For this review, take the finished solid that the model builds, in its own axes (mm). A direction names the side the tool comes from. Coordinates: 2 decimals unless noted, no trailing zeros. Write each loop counter-clockwise with the first axis right and the second up, starting at its lowest first coordinate (ties: lowest second). Pieces come first, ordered by that corner, then holes.
1) We need section C-C on y = -13.5. Write out the cut boundary in (x, z), then the cut area to 3 significant figures.
2) For faces 1 (the face through (-26, -7, -5)), 2 (the face through (-26, -4, -2.5)), 3 (the face through (39.5, -9, 0)), list the 3-axis set-ups (+Z, -Z, +X, -X, +Y, -Y) from which the entire face can be reached by the end or side of a thin tool; tool diameter is ignored.
3) Mouldability with a two-part tool opening along X and no side actions: class faces 4 (the face through (-24.905, -5.456, 4.648)), 5 (the face through (-24.905, -5.456, -4.73)), 6 (the face through (41, -18, -7.52)), 7 (the face through (-42.5, -1, 0)) as pulls with the +X half, pulls with the -X half, needs draft (parallel to the pull), parting line crosses it, or undercut.
4) To check wall thickness, follow line 1 along Y through (x, z) = (-25.5, -3.8); line 2 along Y through (x, z) = (13, -15.5); line 3 along X through (y, z) = (-9.5, 6.5). State the ranges of each line that lie inside material, in increasing order.
5) We need section A-A on y = -19.1. Write out the cut boundary in (x, z).
6) Insertion check: P1, Ø8.5, axis at y = -12.5, z = -5.5, coming from the -X side; P2, Ø2, axis at x = -25.5, y = -5, coming from the +Z side; P3, Ø3, axis at x = -25.5, y = -6, coming from the -Z side. Each pin has a flat end and moves straight along its axis. Give the tip position at first contact, or say it passes through.
from build123d import *

# Parameters (mm, degrees)
SKETCH1_W                  = 85
SKETCH1_H                  = 48
BOSS_EXTRUDE1_DEPTH        = 3
SKETCH2_W                  = 3
SKETCH2_H                  = 48
BOSS_EXTRUDE2_DEPTH        = 18
M1_6_CLEARANCE_HOLE2_D     = 1.8
SKETCH11_W                 = 15.04
SKETCH11_H                 = 5
CUT_EXTRUDE5_DEPTH         = 91.785461391
SKETCH14_W                 = 10.48
SKETCH14_H                 = 18
CUT_EXTRUDE6_DEPTH         = 88.982952894
FILLET1_R                  = 1
FILLET2_R                  = 1
FILLET3_R                  = 1
FILLET4_R                  = 1
FILLET5_R                  = 1
FILLET6_R                  = 1
SKETCH17_R                 = 23
CUT_EXTRUDE11_DEPTH        = 1
FILLET9_R                  = 1
FILLET10_R                 = 10
FILLET11_R                 = 10
SKETCH18_W                 = 6
SKETCH18_H                 = 4.397787755
SKETCH18_H_2               = 4.357175314
BOSS_EXTRUDE3_DEPTH        = 4
F_1_5_1_5_DIAMETER_HOLE1_D = 1.5


with BuildPart() as part:
    # Sketch1 → Boss-Extrude1 (new body)
    with BuildSketch(Plane(origin=(0, 0, 0), x_dir=(1, 0, 0), z_dir=(0, 1, 0))):
        Rectangle(SKETCH1_W, SKETCH1_H)
    extrude(amount=-BOSS_EXTRUDE1_DEPTH)

    # Sketch2 → Boss-Extrude2 (add)
    with BuildSketch(Plane.XZ.offset(3)):
        with Locations((41, 0)):
            Rectangle(SKETCH2_W, SKETCH2_H)
    extrude(amount=BOSS_EXTRUDE2_DEPTH)

    # M1.6 Clearance Hole2 (through all)
    with Locations(Plane(origin=(0, 0, -24), x_dir=(-1, 0, 0), z_dir=(0, 0, -1))):
        with Locations((-41, -19.1)):
            Hole(M1_6_CLEARANCE_HOLE2_D / 2)

    # Sketch11 → Cut-Extrude5 (cut, through all)
    with BuildSketch(Plane(origin=(42.5, 0, 0), x_dir=(0, 0, -1), z_dir=(1, 0, 0))):
        with Locations((0, -18.5)):
            Rectangle(SKETCH11_W, SKETCH11_H)
    extrude(amount=-CUT_EXTRUDE5_DEPTH, mode=Mode.SUBTRACT)

    # Sketch14 → Cut-Extrude6 (cut, through all)
    with BuildSketch(Plane.ZY.offset(-39.5)):
        with Locations((-18.76, -12)):
            Rectangle(SKETCH14_W, SKETCH14_H)
        with Locations((18.76, -12)):
            Rectangle(SKETCH14_W, SKETCH14_H)
    extrude(amount=-CUT_EXTRUDE6_DEPTH, mode=Mode.SUBTRACT)

    # Fillet1
    fillet1_edges = [part.edges().sort_by_distance(p)[0] for p in [
        (42.5, -21, -10.52),
    ]]
    fillet(fillet1_edges, radius=FILLET1_R)

    # Fillet2
    fillet2_edges = [part.edges().sort_by_distance(p)[0] for p in [
        (42.5, -21, 10.52),
    ]]
    fillet(fillet2_edges, radius=FILLET2_R)

    # Fillet3
    fillet3_edges = [part.edges().sort_by_distance(p)[0] for p in [
        (39.5, -21, -10.52),
    ]]
    fillet(fillet3_edges, radius=FILLET3_R)

    # Fillet4
    fillet4_edges = [part.edges().sort_by_distance(p)[0] for p in [
        (39.5, -21, 10.52),
    ]]
    fillet(fillet4_edges, radius=FILLET4_R)

    # Fillet5
    fillet5_edges = [part.edges().sort_by_distance(p)[0] for p in [
        (42.5, -16, 0),
    ]]
    fillet(fillet5_edges, radius=FILLET5_R)

    # Fillet6
    fillet6_edges = [part.edges().sort_by_distance(p)[0] for p in [
        (39.5, -16, 0),
    ]]
    fillet(fillet6_edges, radius=FILLET6_R)

    # Sketch17 → Cut-Extrude11 (cut)
    with BuildSketch(Plane.XZ.offset(3)):
        with Locations(Location((2.21, 0, 0), (0, 0, 270))):
            Circle(SKETCH17_R)
    extrude(amount=-CUT_EXTRUDE11_DEPTH, mode=Mode.SUBTRACT)

    # Fillet9
    fillet9_edges = [part.edges().sort_by_distance(p)[0] for p in [
        (2.21, -3, 23),
    ]]
    fillet(fillet9_edges, radius=FILLET9_R - 0.0001)  # a hair under: the kernel refuses the full size

    # Fillet10
    fillet10_edges = [part.edges().sort_by_distance(p)[0] for p in [
        (-42.5, -1.5, -24),
    ]]
    fillet(fillet10_edges, radius=FILLET10_R)

    # Fillet11
    fillet11_edges = [part.edges().sort_by_distance(p)[0] for p in [
        (-42.5, -1.5, 24),
    ]]
    fillet(fillet11_edges, radius=FILLET11_R)

    # Sketch18 → Boss-Extrude3 (add)
    with BuildSketch(Plane.XZ.offset(3)):
        with Locations((-25.5, -4.698893877)):
            Rectangle(SKETCH18_W, SKETCH18_H)
        with Locations((-25.5, 4.678587657)):
            Rectangle(SKETCH18_W, SKETCH18_H_2)
    extrude(amount=BOSS_EXTRUDE3_DEPTH)

    # Ø1.5 (1.5) Diameter Hole1 (through all)
    with Locations(Plane.XY.offset(6.857175314)):
        with Locations((-25.5, -5)):
            Hole(F_1_5_1_5_DIAMETER_HOLE1_D / 2)


solid = part.part
Result:
1. outline: (39.5, -13.52) - (42.5, -13.52) - (42.5, 13.52) - (39.5, 13.52) - close
1. area: 81.1 mm2
2. face 1: +Z, -Z, -X, -Y
2. face 2: -X, -Y
2. face 3: +Z, -Z, -Y
3. face 4: undercut
3. face 5: undercut
3. face 6: needs draft
3. face 7: pulls with the -X half
4. line 1: y = -7 to -5.75, -4.25 to 0
4. line 2: y = -2 to 0
4. line 3: x = 39.5 to 42.5
5. outline: (39.5, -13.52) - (40.1, -13.52) - (40.1, -7.52) - (39.5, -7.52) - close; (39.5, 7.52) - (40.1, 7.52) - (40.1, 13.52) - (39.5, 13.52) - close; (41.9, -13.52) - (42.5, -13.52) - (42.5, -7.52) - (41.9, -7.52) - close; (41.9, 7.52) - (42.5, 7.52) - (42.5, 13.52) - (41.9, 13.52) - close
6. P1: stops at x = 39.5
6. P2: stops at z = 6.86
6. P3: stops at z = -6.9
